The model under review builds one solid part; all positions refer to its coordinate system, in mm. Face numbers are marked on the shaded views. A direction names the side the tool comes from. Round coordinates to 2 decimals unless told otherwise and drop trailing zeros. Loops run counter-clockwise (first coordinate to the right, second up) from the corner with the lowest first, then second, coordinate; pieces in that order, holes last. Notation, with made-up numbers: M 10,-19 L 35,-19 A12 cw 35,-4 Z; hole C -1.5,-17.5 d4. An arc over 180 degrees is marked long. Answer in a Markdown table with one row per item. Add a question column.
from build123d import *

# Parameters (mm, degrees)
F0_W     = 50
F0_H     = 50
F0_W_2   = 20
F0_H_2   = 20
F1_DEPTH = 10
F2_W     = 30
F2_H     = 30
F2_W_2   = 20
F2_H_2   = 20
F3_DEPTH = 30
F4_W     = 50
F4_H     = 50
F4_W_2   = 20
F4_H_2   = 20
F5_DEPTH = 10


with BuildPart() as f1:
    # F0 (on Top) → F1 (new body)
    with BuildSketch(Plane.XY):
        with Locations((-21.768434, 10.361008)):
            Rectangle(F0_W, F0_H)
        with Locations((-21.768434, 10.361008)):
            Rectangle(F0_W_2, F0_H_2, mode=Mode.SUBTRACT)
    extrude(amount=F1_DEPTH)

    # F2 (on face) → F3 (join)
    with BuildSketch(Plane(origin=(0, 0, 0), x_dir=(1, 0, 0), z_dir=(0, 0, -1))):
        with Locations((-21.768434, -10.361008)):
            Rectangle(F2_W, F2_H)
        with Locations((-21.768434, -10.361008)):
            Rectangle(F2_W_2, F2_H_2, mode=Mode.SUBTRACT)
    extrude(amount=F3_DEPTH)

    # F4 (on face) → F5 (join)
    with BuildSketch(Plane(origin=(0, 0, -30), x_dir=(1, 0, 0), z_dir=(0, 0, -1))):
        with Locations((-21.598472, -9.984265)):
            Rectangle(F4_W, F4_H)
        with Locations((-21.768434, -10.361008)):
            Rectangle(F4_W_2, F4_H_2, mode=Mode.SUBTRACT)
    extrude(amount=F5_DEPTH)


solid = f1.part
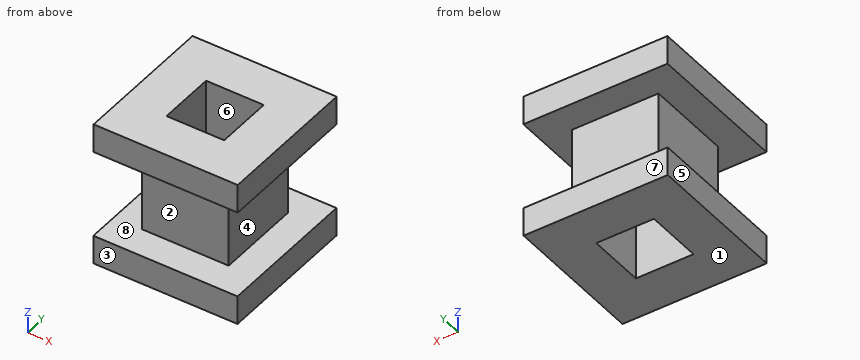
1. Take a section at A-A, the plane x = -13. State the section outline as (y, z) points.
2. To check wall thickness, follow probe 1 along Z at (x, y) = (-43, 4); probe 2 along Y at (x, z) = (-25, -20); probe 3 along X at (y, z) = (16, -11.5). State the ranges of each line that lie inside material, in increasing order.
3. Take a section at C-C, the plane y = -11. State the section outline as (x, z) points.
4. Take a section at D-D, the plane y = -1.5. State the section outline as (x, z) points, and give its area (3 significant figures).
5. Take a section at B-B, the plane z = -34. State the section outline as (x, y) points, and give its area (3 significant figures).
6. Mouldability with a two-part tool opening along Z and no side actions: class the marked faces 1, 2 and 3 as released by +Z, released by -Z, zero draft, split by the parting line, or undercut.
7. For pin 1 Ø16 at (x, z) = (-22.5, -8.5) entering from +Y; pin 2 Ø3 at (x, z) = (-18, 3.5) entering from -Y; pin 3 Ø6 at (x, z) = (-19.5, -22.5) entering from -Y, all flat-tipped, find the tip position at first contact; note any pin that passes through.
8. Machinability: for the marked faces 4, 5, 6, 7 and 8, which of the approach directions +Z, -Z, +X, -X, +Y, -Y give a long, thin tool a straight path to every point of the face, cutting with its end or side? Answer none if there is none.
Check sheet entries:
| question | item | result |
|---|---|---|
| 1 | outline | M -15.02,-40 L 0.36,-40 L 0.36,10 L -14.64,10 L -14.64,0 L -4.64,0 L -4.64,-30 L -15.02,-30 Z; M 20.36,-40 L 34.98,-40 L 34.98,-30 L 25.36,-30 L 25.36,0 L 35.36,0 L 35.36,10 L 20.36,10 Z |
| 2 | probe 1 | z = -40 to -30, 0 to 10 |
| 2 | probe 2 | y = -4.64 to 0.36, 20.36 to 25.36 |
| 2 | probe 3 | x = -36.77 to -31.77, -11.77 to -6.77 |
| 3 | outline | M -46.77,0 L 3.23,0 L 3.23,10 L -46.77,10 Z; M -46.6,-40 L 3.4,-40 L 3.4,-30 L -46.6,-30 Z |
| 4 | outline | M -46.77,0 L -36.77,0 L -36.77,-30 L -46.6,-30 L -46.6,-40 L 3.4,-40 L 3.4,-30 L -6.77,-30 L -6.77,0 L 3.23,0 L 3.23,10 L -46.77,10 Z |
| 4 | area | 1,900 mm^2 |
| 5 | outline | M -46.6,-15.02 L 3.4,-15.02 L 3.4,34.98 L -46.6,34.98 Z; hole M -31.77,0.36 L -11.77,0.36 L -11.77,20.36 L -31.77,20.36 Z |
| 5 | area | 2,100 mm^2 |
| 6 | face 1 | released by -Z |
| 6 | face 2 | undercut |
| 6 | face 3 | zero draft |
| 7 | pin 1 | stops at y = 25.36 |
| 7 | pin 2 | stops at y = -14.64 |
| 7 | pin 3 | stops at y = -4.64 |
| 8 | face 4 | +X, +Y, -Y |
| 8 | face 5 | -Z, -X, +Y, -Y |
| 8 | face 6 | +Z, -Z |
| 8 | face 7 | -Z, +X, -X, +Y |
| 8 | face 8 | none |
